Answer from the drawing. Dimensions are ordinates in mm from the lowest x, y and z of the part. A direction names the side the tool comes from. Coordinates: 2 decimals unless noted, no trailing zeros. Loops run counter-clockwise (first coordinate to the right, second up) from the corner with the lowest first, then second, coordinate; pieces in that order, holes last.
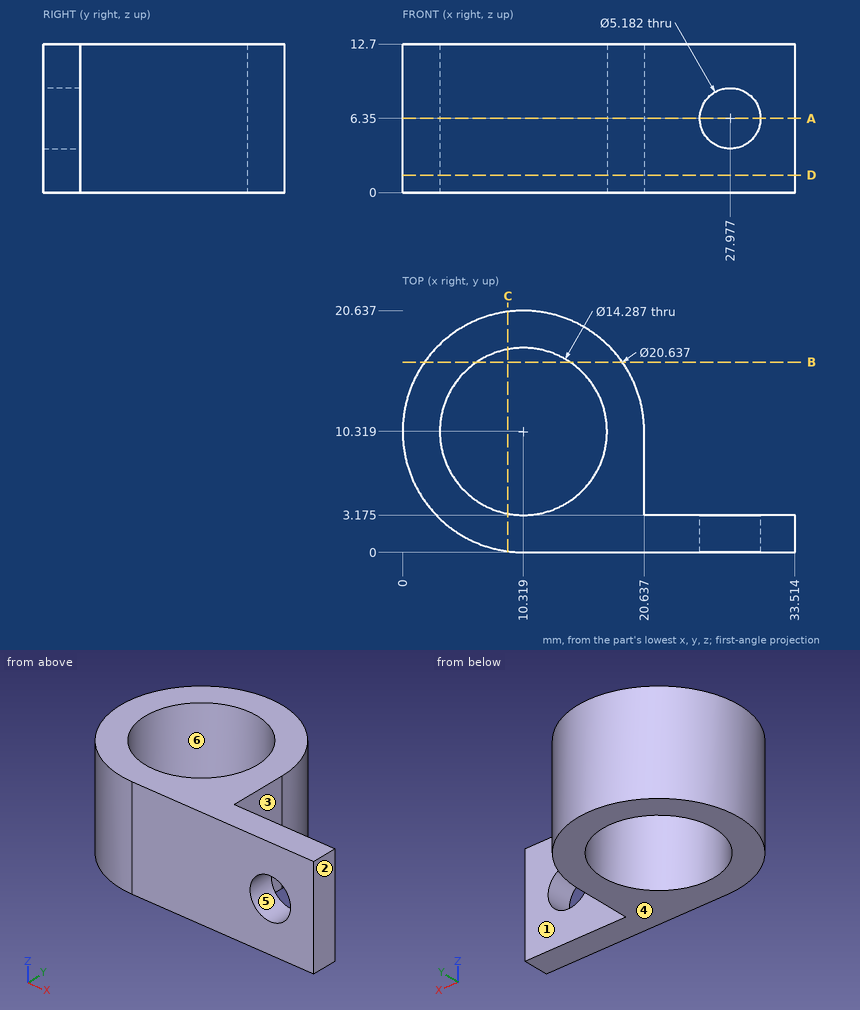
Item 1: A cutting plane is placed at C-C on x = 9. Determine the outline of the cut face in (y, z) (1 decimal).
Numbers:
outline: (0.1, 0) - (3.3, 0) - (3.3, 12.7) - (0.1, 12.7) - close; (17.3, 0) - (20.6, 0) - (20.6, 12.7) - (17.3, 12.7) - close
Item 2: Given pin 1 (5 mm diameter, centred on x = 22, z = 6.5, fed in from +Y) (1 decimal); pin 2 (6.5 mm diameter, centred on x = 24.5, z = 3.5, fed in from +Y) (1 decimal); pin 3 (5 mm diameter, centred on x = 4.5, z = 3, fed in from -Y), each flat-ended and moving along its own axis, determine where each tip first touches the part or whether it passes through.
Numbers:
pin 1: stops at y = 15
pin 2: stops at y = 3.2
pin 3: stops at y = 0.55
Item 3: A cutting plane is placed at A-A on z = 6.35. Determine the outline of the cut face in (x, y) (1 decimal).
Numbers:
outline: (10.3, 0) - (25.4, 0) - (25.4, 3.2) - (20.6, 3.2) - (20.6, 10.3) arc R10.3 ccw (long way) to start; (30.6, 0) - (33.5, 0) - (33.5, 3.2) - (30.6, 3.2) - close; hole circle Ø14.3 at (10.3, 10.3)
Item 4: Find the intervals of material crossed by line 1 along X through (y, z) = (15.75, 8) (1 decimal); line 2 along Y through (x, z) = (21, 11) (1 decimal); line 3 along X through (y, z) = (9.5, 2.25) (1 decimal), in increasing order.
Numbers:
line 1: x = 1.5 to 5.7, 15 to 19.1
line 2: y = 0 to 3.2
line 3: x = 0 to 3.2, 17.4 to 20.6
Item 5: A cutting plane is placed at B-B on y = 16.25. Determine the outline of the cut face in (x, z) (1 decimal), then the cut area to 3 significant figures.
Numbers:
outline: (1.9, 0) - (6.3, 0) - (6.3, 12.7) - (1.9, 12.7) - close; (14.3, 0) - (18.8, 0) - (18.8, 12.7) - (14.3, 12.7) - close
area: 113 mm2
Item 6: Which of the six approach directions +Z, -Z, +X, -X, +Y, -Y give full straight-line access (tool end or side, diameter ignored) to the marked faces 1 and 2?
Numbers:
face 1: +Z, -Z, +X, +Y
face 2: +Z, -Z, +X, +Y, -Y
Item 7: Determine the mould class of the marked faces 3, 4, 5 and 6 for opening direction X: released by +X, released by -X, zero draft, split by the parting line, or undercut.
Numbers:
face 3: released by +X
face 4: zero draft
face 5: undercut
face 6: undercut
Item 8: A cutting plane is placed at D-D on z = 1.5. Determine the outline of the cut face in (x, y) (1 decimal).
Numbers:
outline: (10.3, 0) - (33.5, 0) - (33.5, 3.2) - (20.6, 3.2) - (20.6, 10.3) arc R10.3 ccw (long way) to start; hole circle Ø14.3 at (10.3, 10.3)
